Part model, mm, in its own coordinate system. A direction names the side the tool comes from. Coordinates: 2 decimals unless noted, no trailing zeros. Write each loop counter-clockwise with the first axis right and the second up, starting at its lowest first coordinate (ties: lowest second). Pieces come first, ordered by that corner, then holes. Notation, with made-up numbers: M 66.5,5.5 L 89.5,5.5 A28 cw 89.5,23.5 Z; hole C 86,24 d4. An arc over 180 degrees is marked long. Use a Markdown table: item, result. Add a question column.
Q1. Wall check: L1, parallel to X at y = 82.55, z = 0.3; L2, parallel to X at y = 55.5, z = 153; L3, parallel to Y at x = 140.5, z = 84 (3 decimals). Give the ranges that are in metal, low to high. Write a range as from..to.
Q2. Slice it at A-A on x = 55.5. Write the cut outline in (y, z).
Q3. Mould opens along Y. For faces 1 (the flat face through (133, 0, 81)), 2 (the flat face through (98.23, 6, 82)), 3 (the flat face through (114.154, 82, 6)) say: released by +Y, released by -Y, zero draft, split by the parting line, or undercut.
Q4. Tool access for faces 4 (the flat face through (112.517, 9, 100)), 5 (the flat face through (117.28, 39, 6)), 6 (the flat face through (101.454, 83, 6)): list every direction of +Z, -Z, +X, -X, +Y, -Y with a clear straight run to the whole face (end or side of a thin tool).
Q5. Pin check, flat tips, straight feed: pin 1 Ø18 at (x, z) = (137, 36) entering from +Y; pin 2 Ø1 at (x, y) = (117.5, 94.5) entering from -Z; pin 3 Ø10 at (x, z) = (129, 75.5) entering from +Y; pin 4 Ø1.4 at (x, z) = (114, 64) entering from +Y. Stop position of each tip, or through.
Q6. Slice it at C-C on x = 159.5. Write the cut outline in (y, z) (3 decimals).
from build123d import *

# Parameters (mm, degrees)
BOSS_EXTRUDE2_DEPTH  = 6.35
BOSS_EXTRUDE3_DEPTH  = 6.35
SKETCH3_W            = 1.5875
SKETCH3_H            = 158.75
BOSS_EXTRUDE4_DEPTH  = 6.35
SKETCH4_W            = 12.7
SKETCH4_H            = 6.35
BOSS_EXTRUDE5_DEPTH  = 158.75
SKETCH5_W            = 12.7
SKETCH5_H            = 6.35
BOSS_EXTRUDE6_DEPTH  = 158.75
SKETCH6_W            = 1.5875
SKETCH6_H            = 158.75
BOSS_EXTRUDE7_DEPTH  = 6.35
SKETCH7_W            = 1.5875
SKETCH7_H            = 158.75
BOSS_EXTRUDE8_DEPTH  = 6.35
SKETCH8_W            = 1.5875
SKETCH8_H            = 6.35
BOSS_EXTRUDE9_DEPTH  = 139.7
SKETCH10_W           = 1.5875
SKETCH10_H           = 6.35
BOSS_EXTRUDE10_DEPTH = 139.7
SKETCH11_W           = 12.7
SKETCH11_H           = 12.699759929
BOSS_EXTRUDE11_DEPTH = 101.6
SKETCH12_W           = 101.404934815
SKETCH12_H           = 12.7
BOSS_EXTRUDE12_DEPTH = 6.35
SKETCH13_W           = 101.6
SKETCH13_H           = 12.7
BOSS_EXTRUDE13_DEPTH = 6.35
SKETCH14_W           = 12.7
SKETCH14_H           = 12.7
BOSS_EXTRUDE14_DEPTH = 101.6
SKETCH15_W           = 139.7
SKETCH15_H           = 6.35
BOSS_EXTRUDE15_DEPTH = 63.5
CUT_EXTRUDE1_DEPTH   = 3.175
CUT_EXTRUDE1_DRAFT   = 15
CUT_EXTRUDE3_DEPTH   = 6.35
SKETCH18_W           = 12.7
SKETCH18_H           = 152.4
BOSS_EXTRUDE17_DEPTH = 3.175
SKETCH19_W           = 12.7
SKETCH19_H           = 152.4
BOSS_EXTRUDE18_DEPTH = 3.175
SKETCH20_W           = 12.7
SKETCH20_H           = 152.4
BOSS_EXTRUDE19_DEPTH = 3.175
SKETCH21_W           = 12.7
SKETCH21_H           = 152.4
BOSS_EXTRUDE20_DEPTH = 3.175
SKETCH22_W           = 139.7
SKETCH22_H           = 6.35
BOSS_EXTRUDE21_DEPTH = 3.175
SKETCH23_W           = 139.7
SKETCH23_H           = 12.699759929
BOSS_EXTRUDE22_DEPTH = 3.175
CUT_EXTRUDE4_DEPTH   = 12.7
SKETCH30_W           = 12.7
SKETCH30_H           = 26.035
BOSS_EXTRUDE25_DEPTH = 3.175
SKETCH31_W           = 12.7
SKETCH31_H           = 26.035
BOSS_EXTRUDE26_DEPTH = 3.175
BOSS_EXTRUDE27_DEPTH = 12.7
BOSS_EXTRUDE28_DEPTH = 12.7
SKETCH37_R           = 0.635
BOSS_EXTRUDE29_DEPTH = 7.9375
CUT_EXTRUDE5_START   = -8.4455
SKETCH38_R           = 0.635
CUT_EXTRUDE5_DEPTH   = 8.4455
CUT_EXTRUDE6_START   = -8.4455
SKETCH39_R           = 0.635
CUT_EXTRUDE6_DEPTH   = 8.4455
CUT_EXTRUDE7_START   = -8.4455
SKETCH40_R           = 0.635
CUT_EXTRUDE7_DEPTH   = 8.4455
CUT_EXTRUDE8_START   = -8.4455
SKETCH41_R           = 0.635
CUT_EXTRUDE8_DEPTH   = 8.4455


with BuildPart() as part:
    # Sketch1 → Boss-Extrude2 (new body)
    with BuildSketch(Plane.XY):
        Polygon((0, 0), (215.704934815, 0), (215.704934815, 12.7), (114.104934815, 12.7), (114.104934815, 165.1), (101.404934815, 165.1), (101.404934815, 12.7), (0, 12.7), align=None)
    extrude(amount=BOSS_EXTRUDE2_DEPTH)

    # Sketch2 → Boss-Extrude3 (add)
    with BuildSketch(Plane.XY.offset(6.35)):
        Polygon((101.404934815, 12.7), (101.404934815, 6.35), (102.992434815, 6.35), (102.992434815, 165.1), (101.404934815, 165.1), align=None)
    extrude(amount=BOSS_EXTRUDE3_DEPTH)

    # Sketch3 → Boss-Extrude4 (add)
    with BuildSketch(Plane.XY.offset(6.35)):
        with Locations((113.311184815, 85.725)):
            Rectangle(SKETCH3_W, SKETCH3_H)
    extrude(amount=BOSS_EXTRUDE4_DEPTH)

    # Sketch4 → Boss-Extrude5 (add)
    with BuildSketch(Plane.XY.offset(6.35)):
        with Locations((107.754934815, 3.175)):
            Rectangle(SKETCH4_W, SKETCH4_H)
    extrude(amount=BOSS_EXTRUDE5_DEPTH)

    # Sketch5 → Boss-Extrude6 (add)
    with BuildSketch(Plane(origin=(0, 6.35, 0), x_dir=(1, 0, 0), z_dir=(0, 1, 0))):
        with Locations((107.754934815, -161.925)):
            Rectangle(SKETCH5_W, SKETCH5_H)
    extrude(amount=BOSS_EXTRUDE6_DEPTH)

    # Sketch6 → Boss-Extrude7 (add)
    with BuildSketch(Plane(origin=(0, 0, 158.75), x_dir=(-1, 0, 0), z_dir=(0, 0, -1))):
        with Locations((-102.198684815, 85.725)):
            Rectangle(SKETCH6_W, SKETCH6_H)
    extrude(amount=BOSS_EXTRUDE7_DEPTH)

    # Sketch7 → Boss-Extrude8 (add)
    with BuildSketch(Plane(origin=(0, 0, 158.75), x_dir=(-1, 0, 0), z_dir=(0, 0, -1))):
        with Locations((-113.311184815, 85.725)):
            Rectangle(SKETCH7_W, SKETCH7_H)
    extrude(amount=BOSS_EXTRUDE8_DEPTH)

    # Sketch8 → Boss-Extrude9 (add)
    with BuildSketch(Plane(origin=(0, 0, 152.4), x_dir=(-1, 0, 0), z_dir=(0, 0, -1))):
        with Locations((-113.311184815, 9.525)):
            Rectangle(SKETCH8_W, SKETCH8_H)
    extrude(amount=BOSS_EXTRUDE9_DEPTH)

    # Sketch10 → Boss-Extrude10 (add)
    with BuildSketch(Plane.XY.offset(12.7)):
        with Locations((102.198684815, 9.525)):
            Rectangle(SKETCH10_W, SKETCH10_H)
    extrude(amount=BOSS_EXTRUDE10_DEPTH)

    # Sketch11 → Boss-Extrude11 (add)
    with BuildSketch(Plane.ZY.offset(-101.404934815)):
        with Locations((158.75, 6.349879965)):
            Rectangle(SKETCH11_W, SKETCH11_H)
    extrude(amount=BOSS_EXTRUDE11_DEPTH)

    # Sketch12 → Boss-Extrude12 (add)
    with BuildSketch(Plane.XY.offset(6.35)):
        with Locations((50.702467408, 6.35)):
            Rectangle(SKETCH12_W, SKETCH12_H)
    extrude(amount=BOSS_EXTRUDE12_DEPTH)

    # Sketch13 → Boss-Extrude13 (add)
    with BuildSketch(Plane.XY.offset(6.35)):
        with Locations((164.904934815, 6.35)):
            Rectangle(SKETCH13_W, SKETCH13_H)
    extrude(amount=BOSS_EXTRUDE13_DEPTH)

    # Sketch14 → Boss-Extrude14 (add)
    with BuildSketch(Plane(origin=(114.104934815, 0, 0), x_dir=(0, 0, -1), z_dir=(1, 0, 0))):
        with Locations((-158.75, 6.35)):
            Rectangle(SKETCH14_W, SKETCH14_H)
    extrude(amount=BOSS_EXTRUDE14_DEPTH)

    # Sketch15 → Boss-Extrude15 (add)
    with BuildSketch(Plane(origin=(114.104934815, 0, 0), x_dir=(0, 0, -1), z_dir=(1, 0, 0))):
        with Locations((-82.55, 3.175)):
            Rectangle(SKETCH15_W, SKETCH15_H)
    extrude(amount=BOSS_EXTRUDE15_DEPTH)


with BuildPart() as cut_extrude1_tool:
    # Sketch16 → Cut-Extrude1 (with draft: the straight prism first)
    with BuildSketch(Plane(origin=(0, 6.35, 0), x_dir=(1, 0, 0), z_dir=(0, 1, 0))):
        Polygon((177.604934815, -82.55), (177.604934815, -79.375), (114.104934815, -79.375), (114.104934815, -82.55), (114.104934815, -85.725), (177.604934815, -85.725), align=None)
    extrude(amount=-CUT_EXTRUDE1_DEPTH)
    # Cut-Extrude1: the draft: its side faces are tilted about the plane it starts from
    cut_extrude1_sides = [cut_extrude1_tool.faces().sort_by_distance(p)[0] for p in [
        (177.604934815, 4.7625, 82.55),
        (114.104934815, 4.7625, 82.55),
        (145.854934815, 4.7625, 85.725),
        (145.854934815, 4.7625, 79.375),
    ]]
    draft(cut_extrude1_sides, Plane(origin=(0, 6.35, 0), x_dir=(1, 0, 0), z_dir=(0, 1, 0)), CUT_EXTRUDE1_DRAFT)


with BuildPart() as part_1:
    add(part.part)

    # Cut-Extrude1: cut by cut_extrude1_tool
    add(cut_extrude1_tool.part, mode=Mode.SUBTRACT)

    # Sketch17 → Cut-Extrude3 (cut)
    with BuildSketch(Plane(origin=(0, 0, 0), x_dir=(-1, 0, 0), z_dir=(0, 0, -1))):
        Polygon((-107.803701111, 87.3125), (-112.566201111, 87.3125), (-112.566201111, 82.55), (-112.566201111, 77.784684897), (-107.806516214, 77.784684897), (-103.041201111, 77.784684897), (-103.041201111, 82.55), (-103.041201111, 87.3125), align=None)
    extrude(amount=-CUT_EXTRUDE3_DEPTH, mode=Mode.SUBTRACT)

    # Sketch18 → Boss-Extrude17 (add)
    with BuildSketch(Plane.ZY.offset(-101.404934815)):
        with Locations((6.35, 88.9)):
            Rectangle(SKETCH18_W, SKETCH18_H)
    extrude(amount=BOSS_EXTRUDE17_DEPTH)

    # Sketch19 → Boss-Extrude18 (add)
    with BuildSketch(Plane(origin=(114.104934815, 0, 0), x_dir=(0, 0, -1), z_dir=(1, 0, 0))):
        with Locations((-6.35, 88.9)):
            Rectangle(SKETCH19_W, SKETCH19_H)
    extrude(amount=BOSS_EXTRUDE18_DEPTH)

    # Sketch20 → Boss-Extrude19 (add)
    with BuildSketch(Plane.ZY.offset(-101.404934815)):
        with Locations((158.75, 88.9)):
            Rectangle(SKETCH20_W, SKETCH20_H)
    extrude(amount=BOSS_EXTRUDE19_DEPTH)

    # Sketch21 → Boss-Extrude20 (add)
    with BuildSketch(Plane(origin=(114.104934815, 0, 0), x_dir=(0, 0, -1), z_dir=(1, 0, 0))):
        with Locations((-158.75, 88.9)):
            Rectangle(SKETCH21_W, SKETCH21_H)
    extrude(amount=BOSS_EXTRUDE20_DEPTH)

    # Sketch22 → Boss-Extrude21 (add)
    with BuildSketch(Plane(origin=(114.104934815, 0, 0), x_dir=(0, 0, -1), z_dir=(1, 0, 0))):
        with Locations((-82.55, 9.525)):
            Rectangle(SKETCH22_W, SKETCH22_H)
    extrude(amount=BOSS_EXTRUDE21_DEPTH)

    # Sketch23 → Boss-Extrude22 (add)
    with BuildSketch(Plane.ZY.offset(-101.404934815)):
        with Locations((82.55, 6.349879965)):
            Rectangle(SKETCH23_W, SKETCH23_H)
    extrude(amount=BOSS_EXTRUDE22_DEPTH)

    # Sketch25 → Cut-Extrude4 (cut)
    with BuildSketch(Plane(origin=(0, 0, 0), x_dir=(-1, 0, 0), z_dir=(0, 0, -1))):
        Polygon((-112.566201111, 88.9), (-101.453701111, 88.9), (-101.453701111, 76.2), (-114.153701111, 76.2), (-114.153701111, 88.9), align=None)
    extrude(amount=-CUT_EXTRUDE4_DEPTH, mode=Mode.SUBTRACT)

    # Sketch30 → Boss-Extrude25 (add)
    with BuildSketch(Plane(origin=(117.279934815, 0, 0), x_dir=(0, 0, -1), z_dir=(1, 0, 0))):
        with Locations((-6.35, 86.0425)):
            Rectangle(SKETCH30_W, SKETCH30_H)
    extrude(amount=BOSS_EXTRUDE25_DEPTH)

    # Sketch31 → Boss-Extrude26 (add)
    with BuildSketch(Plane.ZY.offset(-98.229934815)):
        with Locations((6.35, 86.0425)):
            Rectangle(SKETCH31_W, SKETCH31_H)
    extrude(amount=BOSS_EXTRUDE26_DEPTH)

    # Sketch32 → Boss-Extrude27 (add)
    with BuildSketch(Plane(origin=(0, 0, 0), x_dir=(-1, 0, 0), z_dir=(0, 0, -1))):
        Polygon((-120.454934815, 73.025), (-117.279934815, 63.840058945), (-117.279934815, 73.025), align=None)
    extrude(amount=-BOSS_EXTRUDE27_DEPTH)

    # Sketch36 → Boss-Extrude28 (add)
    with BuildSketch(Plane(origin=(0, 0, 0), x_dir=(-1, 0, 0), z_dir=(0, 0, -1))):
        Polygon((-95.054934815, 73.025), (-98.229934815, 63.911198594), (-98.229934815, 73.025), align=None)
    extrude(amount=-BOSS_EXTRUDE28_DEPTH)

    # Sketch37 → Boss-Extrude29 (add)
    with BuildSketch(Plane(origin=(0, 0, 0), x_dir=(-1, 0, 0), z_dir=(0, 0, -1))):
        with Locations(Location((-117.803681111, 82.55, 0), (0, 0, 180))):
            Circle(SKETCH37_R)
        with Locations(Location((-96.803672311, 82.55, 0), (0, 0, 180))):
            Circle(SKETCH37_R)
        with Locations(Location((-96.803672311, 94.5500014, 0), (0, 0, 180))):
            Circle(SKETCH37_R)
        with Locations(Location((-117.803681111, 94.5500014, 0), (0, 0, 180))):
            Circle(SKETCH37_R)
    extrude(amount=BOSS_EXTRUDE29_DEPTH)

    # Sketch38 → Cut-Extrude5 (cut)
    with BuildSketch(Plane(origin=(0, 0, -7.9375), x_dir=(-1, 0, 0), z_dir=(0, 0, -1)).offset(CUT_EXTRUDE5_START)):
        with Locations((-117.803681111, 94.5500014)):
            Circle(SKETCH38_R)
    extrude(amount=CUT_EXTRUDE5_DEPTH, mode=Mode.SUBTRACT)

    # Sketch39 → Cut-Extrude6 (cut)
    with BuildSketch(Plane(origin=(0, 0, -7.9375), x_dir=(-1, 0, 0), z_dir=(0, 0, -1)).offset(CUT_EXTRUDE6_START)):
        with Locations((-96.803672311, 94.5500014)):
            Circle(SKETCH39_R)
    extrude(amount=CUT_EXTRUDE6_DEPTH, mode=Mode.SUBTRACT)

    # Sketch40 → Cut-Extrude7 (cut)
    with BuildSketch(Plane(origin=(0, 0, -7.9375), x_dir=(-1, 0, 0), z_dir=(0, 0, -1)).offset(CUT_EXTRUDE7_START)):
        with Locations((-117.803681111, 82.55)):
            Circle(SKETCH40_R)
    extrude(amount=CUT_EXTRUDE7_DEPTH, mode=Mode.SUBTRACT)

    # Sketch41 → Cut-Extrude8 (cut)
    with BuildSketch(Plane(origin=(0, 0, -7.9375), x_dir=(-1, 0, 0), z_dir=(0, 0, -1)).offset(CUT_EXTRUDE8_START)):
        with Locations((-96.803672311, 82.55)):
            Circle(SKETCH41_R)
    extrude(amount=CUT_EXTRUDE8_DEPTH, mode=Mode.SUBTRACT)


solid = part_1.part
Recorded:
| question | item | result |
|---|---|---|
| 1 | L1 | 95.05..96.17, 97.44..101.45, 114.15..117.17, 118.44..120.45 |
| 1 | L2 | 98.23..102.99, 112.52..117.28 |
| 1 | L3 | 0..3.175 |
| 2 | outline | M 0,0 L 12.7,0 L 12.7,12.7 L 0,12.7 Z; M 0,152.4 L 12.7,152.4 L 12.7,165.1 L 0,165.1 Z |
| 3 | face 1 | released by -Y |
| 3 | face 2 | zero draft |
| 3 | face 3 | undercut |
| 4 | face 4 | +Y |
| 4 | face 5 | +Z, -Z, +X |
| 4 | face 6 | -Z |
| 5 | pin 1 | y = 6.35 |
| 5 | pin 2 | z = 0 |
| 5 | pin 3 | y = 6.35 |
| 5 | pin 4 | y = 12.7 |
| 6 | outline | M 0,0 L 12.7,0 L 12.7,12.7 L 6.35,12.7 L 6.35,79.375 L 3.175,78.524 L 3.175,86.576 L 6.35,85.725 L 6.35,152.4 L 12.7,152.4 L 12.7,165.1 L 0,165.1 Z |
